from build123d import *

# Parameters (mm, degrees)
BOSS_EXTRUDE1_DEPTH = 3.18
FILLET1_R           = 10
SKETCH2_W           = 3.18
SKETCH2_H           = 50
BOSS_EXTRUDE2_DEPTH = 60
FILLET3_R           = 10
FILLET4_R           = 5
SKETCH3_W           = 40.7
SKETCH3_H           = 19.69
CUT_EXTRUDE1_DEPTH  = 170.005332655
SKETCH4_W           = 40.7
SKETCH4_H           = 19.69
CUT_EXTRUDE2_DEPTH  = 3.18
SKETCH5_R           = 1.47
CUT_EXTRUDE3_DEPTH  = 3.18
CIRPATTERN1_COUNT   = 4
SKETCH6_R           = 1.47
CUT_EXTRUDE4_DEPTH  = 3.18
SKETCH8_R           = 1.47
CUT_EXTRUDE6_DEPTH  = 3.18
SKETCH10_W          = 6.5
SKETCH10_H          = 7
CUT_EXTRUDE8_DEPTH  = 3.18
SKETCH11_W          = 6.5
SKETCH11_H          = 7
CUT_EXTRUDE9_DEPTH  = 3.18


with BuildPart() as part:
    # Sketch1 → Boss-Extrude1 (new body)
    with BuildSketch(Plane.XY):
        with BuildLine():
            Line((-105.310889132, 17.5), (-30.310889132, 17.5))
            ThreePointArc((-30.310889132, 17.5), (35, 0), (-30.310889132, -17.5))
            Line((-30.310889132, -17.5), (-105.310889132, -17.5))
            Line((-105.310889132, -17.5), (-105.310889132, 17.5))
        make_face()
    extrude(amount=BOSS_EXTRUDE1_DEPTH)

    # Fillet1
    fillet1_edges = [part.edges().sort_by_distance(p)[0] for p in [
        (-30.310889132, -17.5, 1.59),
        (-30.310889132, 17.5, 1.59),
    ]]
    fillet(fillet1_edges, radius=FILLET1_R)

    # Sketch2 → Boss-Extrude2 (add)
    with BuildSketch(Plane.ZY.offset(105.310889132)):
        with Locations((1.59, 0)):
            Rectangle(SKETCH2_W, SKETCH2_H)
    extrude(amount=BOSS_EXTRUDE2_DEPTH)

    # Fillet3
    # the kernel refuses this fillet: 10 mm, written as the material it adds along each edge
    with BuildSketch(Plane(origin=(-105.310889132, -17.5, 0), x_dir=(0, -1, 0), z_dir=(0, 0, 1))) as fillet3_piece_1:
        with BuildLine():
            CenterArc((10, 9.682458366), FILLET3_R, 180, 75.522487814)
            Line((0, 9.682458366), (-0.2, 9.682458366))
            Line((-0.2, 9.682458366), (-0.2, 0))
            Line((-0.2, 0), (0, -0.2))
            ThreePointArc((0, -0.2), (3.75, -0.2), (7.45, -0.193649167))
            Line((7.45, -0.193649167), (7.5, 0))
        make_face()
    extrude(amount=3.18)
    with BuildSketch(Plane(origin=(-105.310889132, 17.5, 0), x_dir=(0, 1, 0), z_dir=(0, 0, 1))) as fillet3_piece_2:
        with BuildLine():
            CenterArc((10, -9.682458366), FILLET3_R, 104.477512186, 75.522487814)
            Line((0, -9.682458366), (-0.2, -9.682458366))
            Line((-0.2, -9.682458366), (-0.2, 0))
            Line((-0.2, 0), (0, 0.2))
            ThreePointArc((0, 0.2), (3.75, 0.2), (7.45, 0.193649167))
            Line((7.45, 0.193649167), (7.5, 0))
        make_face()
    extrude(amount=3.18)

    # Fillet4
    fillet4_edges = [part.edges().sort_by_distance(p)[0] for p in [
        (-105.310889132, -25, 1.59),
        (-105.310889132, 25, 1.59),
        (-165.310889132, -25, 1.59),
        (-165.310889132, 25, 1.59),
    ]]
    fillet(fillet4_edges, radius=FILLET4_R)

    # Sketch3 → Cut-Extrude1 (cut, through all)
    with BuildSketch(Plane(origin=(0, 0, 0), x_dir=(-1, 0, 0), z_dir=(0, 0, -1))):
        with Locations((10.510889132, 0)):
            Rectangle(SKETCH3_W, SKETCH3_H)
    extrude(amount=-CUT_EXTRUDE1_DEPTH, mode=Mode.SUBTRACT)

    # Sketch4 → Cut-Extrude2 (cut)
    with BuildSketch(Plane(origin=(0, 0, 0), x_dir=(-1, 0, 0), z_dir=(0, 0, -1))):
        with Locations((138.960889132, 0)):
            Rectangle(SKETCH4_W, SKETCH4_H)
    extrude(amount=-CUT_EXTRUDE2_DEPTH, mode=Mode.SUBTRACT)

    # Sketch5 → Cut-Extrude3 (cut)
    with BuildSketch(Plane(origin=(0, 0, 0), x_dir=(-1, 0, 0), z_dir=(0, 0, -1))):
        with Locations((23.68807717, 23.68807717)):
            Circle(SKETCH5_R)
    cut_extrude3 = extrude(amount=-CUT_EXTRUDE3_DEPTH, mode=Mode.SUBTRACT)

    # CirPattern1: Cut-Extrude3 ×4 about axis
    cirpattern1_axis = Axis((0, 0, 0), (0, 0, 1))
    for i in range(1, CIRPATTERN1_COUNT):
        add(cut_extrude3.rotate(cirpattern1_axis, i * 360 / CIRPATTERN1_COUNT), mode=Mode.SUBTRACT)

    # Sketch6 → Cut-Extrude4 (cut)
    with BuildSketch(Plane(origin=(0, 0, 0), x_dir=(-1, 0, 0), z_dir=(0, 0, -1))):
        with Locations((161.310889132, -21)):
            Circle(SKETCH6_R)
        with Locations((111.310889132, -21)):
            Circle(SKETCH6_R)
    cut_extrude4 = extrude(amount=-CUT_EXTRUDE4_DEPTH, mode=Mode.SUBTRACT)

    # Mirror1: Cut-Extrude4 across plane
    add(cut_extrude4.mirror(Plane.ZX), mode=Mode.SUBTRACT)

    # Sketch8 → Cut-Extrude6 (cut)
    with BuildSketch(Plane(origin=(0, 0, 0), x_dir=(-1, 0, 0), z_dir=(0, 0, -1))):
        with Locations((80, 0)):
            Circle(SKETCH8_R)
        with Locations((50, 0)):
            Circle(SKETCH8_R)
    extrude(amount=-CUT_EXTRUDE6_DEPTH, mode=Mode.SUBTRACT)

    # Sketch10 → Cut-Extrude8 (cut)
    with BuildSketch(Plane(origin=(0, 0, 0), x_dir=(-1, 0, 0), z_dir=(0, 0, -1))):
        with Locations((162.560889132, 0)):
            Rectangle(SKETCH10_W, SKETCH10_H)
    extrude(amount=-CUT_EXTRUDE8_DEPTH, mode=Mode.SUBTRACT)

    # Sketch11 → Cut-Extrude9 (cut)
    with BuildSketch(Plane(origin=(0, 0, 0), x_dir=(-1, 0, 0), z_dir=(0, 0, -1))):
        with Locations((-13.089110868, 0)):
            Rectangle(SKETCH11_W, SKETCH11_H)
    extrude(amount=-CUT_EXTRUDE9_DEPTH, mode=Mode.SUBTRACT)


solid = part.part
Model file for the job. Use its own axes, mm. A direction names the side the tool comes from. Round coordinates to 2 decimals unless told otherwise and drop trailing zeros. Order: outer loops, then holes, each group sorted by start corner. A loop starts at its lowest first (then second) coordinate and runs counter-clockwise, first axis right, second up.
(1) Band-saw the part on A-A (x = 0). List the corners of the cut face in (y, z) (3 decimals).
(2) Pin check, flat tips, straight feed: pin 1 (2.5 mm diameter, centred on x = 23.69, y = 23.69, fed in from -Z); pin 2 (1 mm diameter, centred on y = 22.5, z = 1, fed in from +X); pin 3 (1 mm diameter, centred on x = 11.5, z = 2, fed in from -Y); pin 4 (1.6 mm diameter, centred on x = -162, z = 1, fed in from +Y). Stop position of each tip, or through.
(3) Band-saw the part on C-C (x = -90). List the corners of the cut face in (y, z).
(4) Drill centre lines: line 1 (Y direction, x = -150, z = 2.75) (3 decimals); line 2 (X direction, y = 22, z = 2.1); line 3 (Y direction, x = -92, z = 2.5). Where is each one in solid material? Low to high.
(5) 3-axis set-ups, long thin cutter, end or side, ignore diameter. For faces 1 (the face through (-67, 0, 0)), 2 (the face through (-31.153, -18.553, 1.612)), 3 (the face through (-100.692, 18.877, 1.568)): which of +Z, -Z, +X, -X, +Y, -Y reach the whole face in a straight line?
(6) Band-saw the part on D-D (y = -29.5). List the corners of the cut face in (x, z).
(7) Band-saw the part on B-B (x = -130.5). List the corners of the cut face in (y, z) (3 decimals).
(8) Pull direction X, two halves, no side cores. Call faces 4 (the face through (-163.885, -23.496, 1.612)), 5 (the face through (-67, 0, 3.18)), 6 (the face through (-31.267, 18.497, 1.612)): released by +X, released by -X, zero draft, split by the parting line, or undercut.
Verdict:
1. outline: (-35, 0) - (-9.845, 0) - (-9.845, 3.18) - (-35, 3.18) - close; (9.845, 0) - (35, 0) - (35, 3.18) - (9.845, 3.18) - close
2. pin 1: passes through
2. pin 2: stops at x = 27.22
2. pin 3: stops at y = -33.23
2. pin 4: stops at y = 24.92
3. outline: (-17.5, 0) - (17.5, 0) - (17.5, 3.18) - (-17.5, 3.18) - close
4. line 1: y = -25 to -9.845, 9.845 to 25
4. line 2: x = -164.89 to -162.39, -160.23 to -112.39, -110.23 to -103.98, -27.22 to 27.22
4. line 3: y = -17.5 to 17.5
5. face 1: -Z, +X, -X, +Y, -Y
5. face 2: +Z, -Z, -Y
5. face 3: +Z, -Z, +Y
6. outline: (-18.83, 0) - (18.83, 0) - (18.83, 3.18) - (-18.83, 3.18) - close
7. outline: (-25, 0) - (-9.845, 0) - (-9.845, 3.18) - (-25, 3.18) - close; (9.845, 0) - (25, 0) - (25, 3.18) - (9.845, 3.18) - close
8. face 4: released by -X
8. face 5: zero draft
8. face 6: undercut
